```python
from build123d import *

# Parameters (mm, degrees)
F0_W     = 80
F0_H     = 80
F1_DEPTH = 800
F2_W     = 280
F2_H     = 280
F3_DEPTH = 6
F4_SIZE  = 40
F5_R     = 5


with BuildPart() as f1:
    # F0 (on Top) → F1 (new body)
    with BuildSketch(Plane.XY):
        Rectangle(F0_W, F0_H)
    extrude(amount=F1_DEPTH)

    # F2 (on face) → F3 (join)
    with BuildSketch(Plane(origin=(0, 0, 0), x_dir=(1, 0, 0), z_dir=(0, 0, -1))):
        Rectangle(F2_W, F2_H)
    extrude(amount=F3_DEPTH)

    # F4
    f4_edges = [f1.edges().sort_by_distance(p)[0] for p in [
        (140, -140, -3),
        (140, 140, -3),
        (-140, 140, -3),
        (-140, -140, -3),
    ]]
    chamfer(f4_edges, length=F4_SIZE)

    # F5
    f5_edges = [f1.edges().sort_by_distance(p)[0] for p in [
        (140, -100, -3),
        (100, -140, -3),
        (140, 100, -3),
        (100, 140, -3),
        (-100, 140, -3),
        (-140, 100, -3),
        (-100, -140, -3),
        (-140, -100, -3),
    ]]
    fillet(f5_edges, radius=F5_R)


solid = f1.part
```
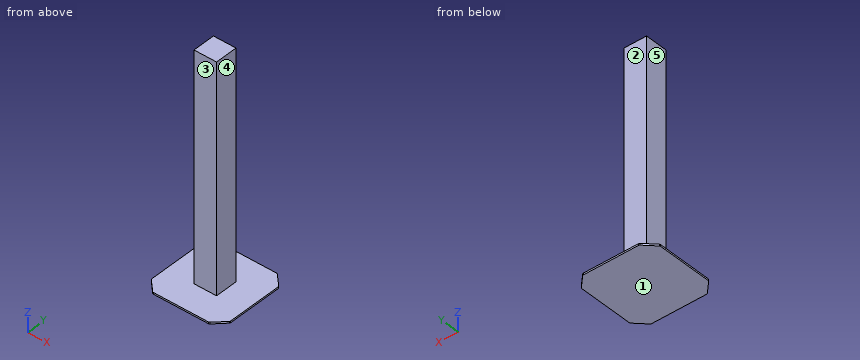
CAD build for the part. Positions are in the model's coordinates, mm. Face numbers are marked on the shaded views. A direction names the side the tool comes from. Round coordinates to 2 decimals unless told otherwise and drop trailing zeros. Order: outer loops, then holes, each group sorted by start corner. A loop starts at its lowest first (then second) coordinate and runs counter-clockwise, first axis right, second up.
Item 1: Saw through at A-A on y = 17.5. Write the cut outline in (x, z).
Item 2: Tool access for the marked faces 1, 2, 3, 4 and 5: list every direction of +Z, -Z, +X, -X, +Y, -Y with a clear straight run to the whole face (end or side of a thin tool).
Item 3: Saw through at C-C on z = 585. Write the cut outline in (x, y), then the cut area to 3 significant figures.
Item 4: Probe line 1 along Z through (x, y) = (84.5, -48); line 2 along Y through (x, z) = (-1, 247). List the from-to ranges inside material, lowest first.
Item 5: Pin check, flat tips, straight feed: pin 1 (8 mm diameter, centred on y = 22, z = 169.5, fed in from -X); pin 2 (24 mm diameter, centred on y = 17, z = 509.5, fed in from +X); pin 3 (1.5 mm diameter, centred on x = 100, y = 48, fed in from +Z). Stop position of each tip, or through.
Item 6: Saw through at D-D on y = -81.5. Write the cut outline in (x, z), then the cut area to 3 significant figures.
Reported:
1. outline: (-140, -6) - (140, -6) - (140, 0) - (40, 0) - (40, 800) - (-40, 800) - (-40, 0) - (-140, 0) - close
2. face 1: -Z, +X, -X, +Y, -Y
2. face 2: +Z, +X, -X, +Y
2. face 3: +Z, +X, -X, -Y
2. face 4: +Z, +X, +Y, -Y
2. face 5: +Z, -X, +Y, -Y
3. outline: (-40, -40) - (40, -40) - (40, 40) - (-40, 40) - close
3. area: 6,400 mm2
4. line 1: z = -6 to 0
4. line 2: y = -40 to 40
5. pin 1: stops at x = -40
5. pin 2: stops at x = 40
5. pin 3: stops at z = 0
6. outline: (-140, -6) - (140, -6) - (140, 0) - (-140, 0) - close
6. area: 1,680 mm2
